Verification items for the finished model (mm, model axes). A direction names the side the tool comes from. Round coordinates to 2 decimals unless told otherwise and drop trailing zeros. Order: outer loops, then holes, each group sorted by start corner. A loop starts at its lowest first (then second) coordinate and runs counter-clockwise, first axis right, second up. Notation, with made-up numbers: M -27.75,-24.5 L 4.25,-24.5 A15 cw 4.25,-16.5 Z; hole C 2,85.25 d8. An arc over 180 degrees is marked long. Use one line per item in the form item = value. Start each with the question number.
Item 1: Cross-section at C-C on y = 146. Enter the section's corners in (x, z), then the cut area to 3 significant figures.
Item 2: Thickness scan on probe 1 along Z at (x, y) = (12, -257); probe 2 along X at (y, z) = (240, -18.6). Record the ranges inside material, lowest first. Write a range as [from, to].
Item 3: Release check for a two-part mould opening along X. For faces 1 (the flat face through (-19, 280, 0)), 2 (the flat face through (-18, -5, 0)), 3 (the flat face through (18, 14, 0)), 4 (the flat face through (-20, -6, 0)) record: +X half, -X half, draft (parallel to the pull), parting line (faces both ways), or undercut.
Item 4: Cross-section at B-B on z = -2. Enter the section's corners in (x, y), then the cut area to 3 significant figures.
Item 5: Tool access check on faces 5 (the flat face through (0, -4, 18)), 6 (the flat face through (0, -280, 19)). Record the directions out of +Z, -Z, +X, -X, +Y, -Y that give a thin tool (end or side, any length) a straight path to the whole face; none if there is none.
Item 6: Go/stop test with flat-tipped pins: pin 1 Ø5.5 at (x, y) = (0, 0) entering from -Z; pin 2 Ø4 at (x, y) = (0, -240) entering from -Z; pin 3 Ø10 at (x, z) = (8.5, 14) entering from -Y. Record where each tip stops, or that it passes through.
Item 7: Cross-section at A-A on x = -12. Enter the section's corners in (y, z), then the cut area to 3 significant figures.
from build123d import *

# Parameters (mm, degrees)
F2_W            = 40
F2_H            = 40
F3_DEPTH        = 300
F4_R            = 3
F5_T            = -2
F7_DEPTH        = 40.001
F9_DEPTH        = 40.001
F11_D           = 3.5
F11_CSINK_D     = 6
F11_CSINK_ANGLE = 90


with BuildPart() as f3:
    # F2 (on Front) → F3 (new body, symmetric)
    with BuildSketch(Plane.XZ):
        Rectangle(F2_W, F2_H)
    extrude(amount=F3_DEPTH, both=True)

    # F4
    f4_edges = [f3.edges().sort_by_distance(p)[0] for p in [
        (20, 0, 20),
        (-20, 0, 20),
        (20, 0, -20),
        (-20, 0, -20),
    ]]
    fillet(f4_edges, radius=F4_R)

    # F5
    f5_openings = [f3.faces().sort_by_distance(p)[0] for p in [
        (0, -300, 0),
        (0, 300, 0),
    ]]
    offset(amount=F5_T, openings=f5_openings)

    # F6 (on face) → F7 (cut, through all)
    with BuildSketch(Plane(origin=(-20, 0, 0), x_dir=(0, -1, 0), z_dir=(-1, 0, 0))):
        Polygon((-300, 20), (-300, -20), (-260, -20), align=None)
    extrude(amount=-F7_DEPTH, mode=Mode.SUBTRACT)

    # F8 (on face) → F9 (cut, through all)
    with BuildSketch(Plane.XY.offset(20)):
        Polygon((20, -300), (20, -260), (-20, -300), align=None)
    extrude(amount=-F9_DEPTH, mode=Mode.SUBTRACT)

    # F11 (through all)
    with Locations(Plane(origin=(0, 0, -20), x_dir=(1, 0, 0), z_dir=(0, 0, -1))):
        with Locations((0, 240), (0, 160), (0, 80), (0, 0), (0, -80), (0, -160), (0, -240)):
            CounterSinkHole(F11_D / 2, F11_CSINK_D / 2, counter_sink_angle=F11_CSINK_ANGLE)


solid = f3.part
Output values:
q1.outline = M -20,-17 A3 ccw -17,-20 L 17,-20 A3 ccw 20,-17 L 20,17 A3 ccw 17,20 L -17,20 A3 ccw -20,17 Z; hole M -18,-17 A1 ccw -17,-18 L 17,-18 A1 ccw 18,-17 L 18,17 A1 ccw 17,18 L -17,18 A1 ccw -18,17 Z
q1.area = 297 mm2
q2.probe_1 = [-20, -18], [18, 20]
q2.probe_2 = [-19.54, -1.75], [1.75, 19.54]
q3.face_1 = draft
q3.face_2 = undercut
q3.face_3 = undercut
q3.face_4 = -X half
q4.outline = M -20,-300 L -18,-298 L -18,278 L -20,278 Z; M 18,-262 L 20,-260 L 20,278 L 18,278 Z
q4.area = 2,230 mm2
q5.face_5 = +Y, -Y
q5.face_6 = +Z, -Z, +X, -Y
q6.pin_1 = -19.75
q6.pin_2 = -19
q6.pin_3 = -274.5
q7.outline = M -292,-20 L 260,-20 L 262,-18 L -292,-18 Z; M -292,18 L 298,18 L 300,20 L -292,20 Z
q7.area = 2,290 mm2
